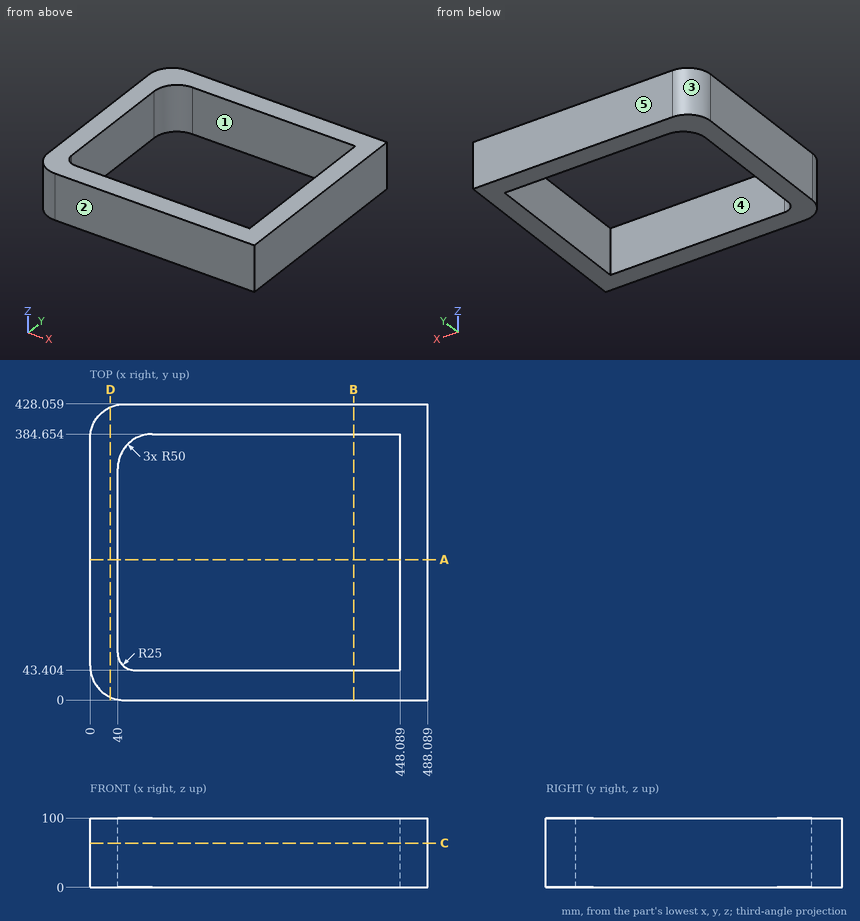
Study the drawing (mm; zero at the part's minimum x, y, z) and answer. A direction names the side the tool comes from. Coordinates: 2 decimals unless noted, no trailing zeros. Loops run counter-clockwise (first coordinate to the right, second up) from the corner with the lowest first, then second, coordinate; pieces in that order, holes last. Notation, with made-up numbers: (28.5, -11) -> (58.5, -11) arc R36 cw to (58.5, 28) -> close; hole circle Ø5 at (-35, 9). An arc over 180 degrees is marked (long way). Write item = value, one per line. Start each with the question number.
1) For the marked faces 1 and 2, determine the directions among +Z, -Z, +X, -X, +Y, -Y from which every point of the face is accessible in a straight line to the end or side of a thin tool.
2) The part is cut by section B-B, the plane x = 381. Determine the outline of the cut face in (y, z) (1 decimal), plus the area to 3 significant figures.
3) The part is cut by section A-A, the plane y = 203. Determine the outline of the cut face in (x, z).
4) Find the intervals of material crossed by L1, parallel to Y at x = 438, z = 85.5 (1 decimal); L2, parallel to X at y = 125, z = 43; L3, parallel to Y at x = 88, z = 64 (1 decimal), in increasing order. Write a range as from..to.
5) The part is cut by section D-D, the plane x = 29.5. Determine the outline of the cut face in (y, z) (1 decimal).
6) The part is cut by section C-C, the plane z = 64. Determine the outline of the cut face in (x, y) (1 decimal), plus the area to 3 significant figures.
7) The mould has two halves that part along X. Classify the marked faces 3, 4 and 5: pulls with the +X half, pulls with the -X half, needs draft (parallel to the pull), parting line crosses it, or undercut.
Result:
q1.face_1 = +Z, -Z
q1.face_2 = +Z, -Z, +X, -X, -Y
q2.outline = (0, 0) -> (43.4, 0) -> (43.4, 100) -> (0, 100) -> close; (384.7, 0) -> (428.1, 0) -> (428.1, 100) -> (384.7, 100) -> close
q2.area = 8,680 mm²
q3.outline = (0, 0) -> (40, 0) -> (40, 100) -> (0, 100) -> close; (448.09, 0) -> (488.09, 0) -> (488.09, 100) -> (448.09, 100) -> close
q4.L1 = 0..43.4, 384.7..428.1
q4.L2 = 0..40, 448.09..488.09
q4.L3 = 0..43.4, 384.6..428.1
q5.outline = (4.4, 0) -> (423.7, 0) -> (423.7, 100) -> (4.4, 100) -> close
q6.outline = (0, 50) arc R50 ccw to (50, 0) -> (488.1, 0) -> (488.1, 428.1) -> (50, 428.1) arc R50 ccw to (0, 378.1) -> close; hole (40, 68.4) arc R25 ccw to (65, 43.4) -> (448.1, 43.4) -> (448.1, 384.7) -> (90, 384.7) arc R50 ccw to (40, 334.7) -> close
q6.area = 69,300 mm²
q7.face_3 = pulls with the -X half
q7.face_4 = undercut
q7.face_5 = needs draft
